```python
from build123d import *

# Parameters (mm, degrees)
F1_DEPTH = 15
F2_R     = 10
F3_DEPTH = 25


with BuildPart() as f1:
    # F0 (on Front) → F1 (new body)
    with BuildSketch(Plane.XZ):
        with BuildLine():
            ThreePointArc((-20, 75), (0, 55), (20, 75))
            ThreePointArc((20, 75), (0, 95), (-20, 75))
        make_face()
        with BuildLine():
            ThreePointArc((-20, 0), (0, 20), (20, 0))
            Line((20, 0), (20, 75))
            ThreePointArc((20, 75), (0, 55), (-20, 75))
            Line((-20, 75), (-20, 0))
        make_face()
        with BuildLine():
            ThreePointArc((-20, 0), (0, -20), (20, 0))
            ThreePointArc((20, 0), (0, 20), (-20, 0))
        make_face()
    extrude(amount=F1_DEPTH)

    # F2 (on face) → F3 (cut)
    with BuildSketch(Plane.XZ.offset(15)):
        with Locations((0, 75)):
            Circle(F2_R)
        Circle(F2_R)
    extrude(amount=-F3_DEPTH, mode=Mode.SUBTRACT)


solid = f1.part
```
Work out the finished part from the listing and answer in its coordinate system (mm). Give positions to 0.01 mm unless a question says otherwise; leave off trailing zeros. Loops run counter-clockwise (first coordinate to the right, second up) from the corner with the lowest first, then second, coordinate; pieces in that order, holes last. Notation, with made-up numbers: (50.25, -8.75) -> (106.25, -8.75) arc R21 cw to (106.25, 11.25) -> close; hole circle Ø8 at (85, 73). An arc over 180 degrees is marked (long way). Use CSV: the item, a comma, the result in double quotes.
1. The mould has two halves that part along X. Classify faces 1 (the cylindrical face through (-2.17, -7.6, -9.76)), 2 (the flat face through (0, -15, 38)), 3 (the cylindrical face through (0, -7, 95)): +X half, -X half, draft (parallel to the pull), parting line (faces both ways), or undercut.
Found:
face 1,"undercut"
face 2,"draft"
face 3,"parting line"
2. Flat-ended cylindrical pins translate along their axes: pin 1 Ø3 at (x, y) = (-8, -8.5) entering from +Z; pin 2 Ø8 at (x, y) = (-14.5, -7) entering from -Z; pin 3 Ø2 at (x, y) = (-11, -13) entering from +Z. Find the tip coordinate at first contact, or state that the pin passes through.
Found:
pin 1,"z = 93.91"
pin 2,"z = -17.02"
pin 3,"z = 92.32"
3. The part is cut by section B-B (z = 71.5). Write down the section's boundary in (x, y), then the cut area to 3 significant figures.
Found:
outline,"(-20, -15) -> (-9.37, -15) -> (-9.37, 0) -> (-20, 0) -> close; (9.37, -15) -> (20, -15) -> (20, 0) -> (9.37, 0) -> close"
area,"319 mm^2"
4. The part is cut by section D-D (x = 5.5). Write down the section's boundary in (y, z).
Found:
outline,"(-15, -19.23) -> (0, -19.23) -> (0, -8.35) -> (-15, -8.35) -> close; (-15, 8.35) -> (0, 8.35) -> (0, 66.65) -> (-15, 66.65) -> close; (-15, 83.35) -> (0, 83.35) -> (0, 94.23) -> (-15, 94.23) -> close"
5. The part is cut by section A-A (x = 0). Write down the section's boundary in (y, z).
Found:
outline,"(-15, -20) -> (0, -20) -> (0, -10) -> (-15, -10) -> close; (-15, 10) -> (0, 10) -> (0, 65) -> (-15, 65) -> close; (-15, 85) -> (0, 85) -> (0, 95) -> (-15, 95) -> close"
6. Straight lines are drawn through the part: line 1 (Z direction, x = 0, y = -11.5); line 2 (Z direction, x = 3, y = -3.5); line 3 (X direction, y = -4, z = -7) (3 decimals). For each, find the intervals that lie inside material, in ascending order.
Found:
line 1,"-20 to -10, 10 to 65, 85 to 95"
line 2,"-19.77 to -9.54, 9.54 to 65.46, 84.54 to 94.77"
line 3,"-18.735 to -7.141, 7.141 to 18.735"
7. The part is cut by section C-C (y = -5). Write down the section's boundary in (x, z), then the cut area to 3 significant figures.
Found:
outline,"(-20, 0) arc R20 ccw to (20, 0) -> (20, 75) arc R20 ccw to (-20, 75) -> close; hole circle Ø20 at (0, 0); hole circle Ø20 at (0, 75)"
area,"3,630 mm^2"
